from build123d import *

# Parameters (mm, degrees)
F0_W     = 140
F0_H     = 40
F1_DEPTH = 3


with BuildPart() as f1:
    # F0 (on Right) → F1 (new body)
    with BuildSketch(Plane.YZ):
        with Locations((-70, 0)):
            Rectangle(F0_W, F0_H)
        with BuildLine():
            ThreePointArc((-130, -14.5), (-132.5, -12), (-130, -9.5))
            Line((-130, -9.5), (-10, -9.5))
            ThreePointArc((-10, -9.5), (-7.5, -12), (-10, -14.5))
            Line((-10, -14.5), (-130, -14.5))
        make_face(mode=Mode.SUBTRACT)
        with BuildLine():
            ThreePointArc((-130, 9.5), (-132.5, 12), (-130, 14.5))
            Line((-130, 14.5), (-10, 14.5))
            ThreePointArc((-10, 14.5), (-7.5, 12), (-10, 9.5))
            Line((-10, 9.5), (-130, 9.5))
        make_face(mode=Mode.SUBTRACT)
    extrude(amount=F1_DEPTH)


solid = f1.part
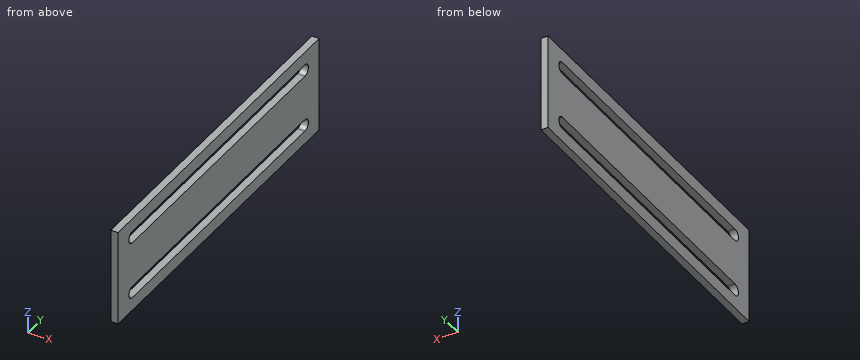
Could you check a few things on this model? Use its own coordinates, in mm. Give positions to 0.01 mm unless a question says otherwise; leave off trailing zeros. Loops run counter-clockwise (first coordinate to the right, second up) from the corner with the lowest first, then second, coordinate; pieces in that order, holes last. Notation, with made-up numbers: (69, -16.75) -> (110, -16.75) arc R35 ccw to (110, 15.25) -> close; hole circle Ø8 at (61.25, 80). An arc over 180 degrees is marked (long way). Answer as CSV lines item,"result". Start each with the question number.
(1) If we section it at A-A on y = -12.5: Write out the boundary of the cut face in (x, z).
(2) If we section it at B-B on z = -12: Write out the boundary of the cut face in (x, y), then the cut area to 3 significant figures.
(3) I need wall thicknesses on probe 1 along Z at (x, y) = (0.6, -58.5); probe 2 along Z at (x, y) = (2.35, -131); probe 3 along Y at (x, z) = (1.7, -11). Which ranges of each line are inside material? Lowest first, please.
(4) If we section it at C-C on x = 0.55: Write out the boundary of the cut face in (y, z), then the cut area to 3 significant figures.
Computed:
1,outline,"(0, -20) -> (3, -20) -> (3, -14.5) -> (0, -14.5) -> close; (0, -9.5) -> (3, -9.5) -> (3, 9.5) -> (0, 9.5) -> close; (0, 14.5) -> (3, 14.5) -> (3, 20) -> (0, 20) -> close"
2,outline,"(0, -140) -> (3, -140) -> (3, -132.5) -> (0, -132.5) -> close; (0, -7.5) -> (3, -7.5) -> (3, 0) -> (0, 0) -> close"
2,area,"45.0 mm2"
3,probe 1,"z = -20 to -14.5, -9.5 to 9.5, 14.5 to 20"
3,probe 2,"z = -20 to -14.29, -9.71 to 9.71, 14.29 to 20"
3,probe 3,"y = -140 to -132.29, -7.71 to 0"
4,outline,"(-140, -20) -> (0, -20) -> (0, 20) -> (-140, 20) -> close; hole (-130, -14.5) -> (-10, -14.5) arc R2.5 ccw to (-10, -9.5) -> (-130, -9.5) arc R2.5 ccw to start; hole (-130, 9.5) -> (-10, 9.5) arc R2.5 ccw to (-10, 14.5) -> (-130, 14.5) arc R2.5 ccw to start"
4,area,"4,360 mm2"
